Autodesk Inventor part; units mm, degrees
ref_plane "作業平面1" through (0, 0, -7.2) normal (0, 0, 1) x (1, 0, 0)
ref_plane "YZ Plane" through (0, 0, 0) normal (1, 0, 0) x (0, 1, 0)
ref_plane "XZ Plane" through (0, 0, 0) normal (0, 1, 0) x (-1, 0, 0)
sketch "スケッチ1" plane through (0, 0, 0) normal (0, 0, 1) x (1, 0, 0)
  circle A0 centre (0, 0) radius 2.5
  dimension "d0" = 5
extrude "押し出し1" add sketch "スケッチ1" along normal blind 18.2
sketch "スケッチ2" plane through (0, 0, 0) normal (0, 0, -1) x (-1, 0, 0)
  circle A0 centre (0, 0) radius 2.5
  circle A1 centre (0, 0) radius 7.5
  dimension "d3" = 15
extrude "押し出し2" add sketch "スケッチ2" against normal blind 4.4
sketch "スケッチ3" plane through (0, 0, 0) normal (0, 0, -1) x (-1, 0, 0)
  circle A0 centre (0, 0) radius 7.5
  circle A1 centre (0, 0) radius 21.05
  dimension "d6" = 42.1
extrude "押し出し3" add sketch "スケッチ3" along normal blind 67 contours A0 | A1
ref_plane "作業平面1" through (0, 0, -7.2) normal (0, 0, 1) x (1, 0, 0)
sketch "スケッチ6" plane through (0, 0, -7.2) normal (0, 0, 1) x (1, 0, 0)
  circle A0 centre (0, 0) radius 23.5
  dimension "d14" = 47
extrude "押し出し5" add sketch "スケッチ6" against normal blind 34
sketch "スケッチ7" plane through (0, 0, 0) normal (0, 0, 1) x (1, 0, 0)
  circle A0 centre (0, 14.5) radius 0.9915
  circle A1 centre (0, 0) radius 2.5
  dimension "d17" = 14.5
hole "穴1" at (0, 14.5, 0) direction (0, 0, -1) diameter 3.242 depth 8 tip angle 118
pattern_circular "放射状パターン1" count 2 over 360 about axis through (0, 0, 0) along (0, 0, 1) of "穴1"
fillet "フィレット1" radius 2 1 edges at (21.05, 0, 0)
fillet "フィレット2" radius 2 2 edges at (-23.5, 0, -7.2) (-23.5, 0, -41.2)
fillet "フィレット3" radius 2 1 edges at (21.05, 0, -67)
properties part number "775"
CAD build for the part. Positions are in the model's coordinates, mm. A direction names the side the tool comes from. Give positions to 0.01 mm unless a question says otherwise; leave off trailing zeros. Loops run counter-clockwise (first coordinate to the right, second up) from the corner with the lowest first, then second, coordinate; pieces in that order, holes last. Notation, with made-up numbers: M 69,-25 L 127,-25 A16 ccw 127,4 Z; hole C 31.25,15 d4. An arc over 180 degrees is marked long. Write each question's results on one line, items separated by ' | '.
Q1. Band-saw the part on B-B on z = -49. Write the cut outline in (x, y), and give its area (3 significant figures).
Geometry check:
outline: C 0,0 d42.1 | area: 1,390 mm²
Q2. Flat gauge pins, fed straight in: P1, Ø21.5, axis at x = -1, y = -8, coming from the +Z side; P2, Ø5, axis at x = 4, z = 4.5, coming from the -Y side; P3, Ø1.5, axis at y = -17.5, z = -10.5, coming from the -X side; P4, Ø19, axis at x = -8.5, y = -9.5, coming from the +Z side. Where does each tip first touch, or does it go through?
Geometry check:
P1: stops at z = 18.2 | P2: stops at y = -7.35 | P3: stops at x = -16.48 | P4: stops at z = 4.4
Q3. Mould opens along Y. For faces 4 (the face through (0, 0, 18.2)), 5 (the face through (0.621, 13.003, -4.056)), 6 (the face through (0.085, 14.231, -8.805)), 7 (the face through (-20.08, -6.32, -4.56)) say: pulls with the +Y half, pulls with the -Y half, needs draft (parallel to the pull), parting line crosses it, or undercut.
Geometry check:
face 4: needs draft | face 5: undercut | face 6: undercut | face 7: parting line crosses it
Q4. Probe probe 1 along Z at (x, y) = (8.5, -3.5); probe 2 along Y at (x, z) = (-1, -30.5); probe 3 along X at (y, z) = (14.5, -2.5). List the from-to ranges inside material, lowest first.
Geometry check:
probe 1: z = -67 to 0 | probe 2: y = -23.48 to 23.48 | probe 3: x = -15.26 to -1.62, 1.62 to 15.26
Q5. Band-saw the part on A-A on y = 0. Write the cut outline in (x, z).
Geometry check:
outline: M -23.5,-39.2 A2 ccw -21.5,-41.2 L -21.05,-41.2 L -21.05,-65 A2 ccw -19.05,-67 L 19.05,-67 A2 ccw 21.05,-65 L 21.05,-41.2 L 21.5,-41.2 A2 ccw 23.5,-39.2 L 23.5,-9.2 A2 ccw 21.5,-7.2 L 21.05,-7.2 L 21.05,-2 A2 ccw 19.05,0 L 7.5,0 L 7.5,4.4 L 2.5,4.4 L 2.5,18.2 L -2.5,18.2 L -2.5,4.4 L -7.5,4.4 L -7.5,0 L -19.05,0 A2 ccw -21.05,-2 L -21.05,-7.2 L -21.5,-7.2 A2 ccw -23.5,-9.2 Z
Q6. Which spindle directions (+Z, -Z, +X, -X, +Y, -Y) get a long thin tool onto all of the face, cutting with end or side? Do faces 1 (the face through (16, -14, -41.2)), 2 (the face through (7.493, 0.33, 2.169)), 3 (the face through (0, 0, -67)). Say none if no direction does.
Geometry check:
face 1: -Z | face 2: +Z | face 3: -Z, +X, -X, +Y, -Y
